Could you check a few things on this drawing? It's one solid part, dimensions in mm from its lowest x, y, z. Round coordinates to 2 decimals unless told otherwise and drop trailing zeros. Write each loop counter-clockwise with the first axis right and the second up, starting at its lowest first coordinate (ties: lowest second). Pieces come first, ordered by that corner, then holes. Notation, with made-up numbers: (48, 34.5) - (105, 34.5) arc R21 ccw to (105, 48.5) - close; hole circle Ø9 at (45.25, -1). An arc over 180 degrees is marked (long way). One line per question, with ' | ' between items. Start each with the question number.
(1) Imagine slicing it at C-C (z = 6.75). Write out the boundary of the cut face in (x, y), plus the area to 3 significant figures.
(2) Will these pins go through, and if not, where does the flat tip stop? pin 1 (1.5 mm diameter, centred on y = 6.5, z = 4, fed in from -X); pin 2 (4 mm diameter, centred on y = 5, z = 3.5, fed in from +X); pin 3 (3.5 mm diameter, centred on x = 4, y = 4, fed in from -Z).
(3) Imagine slicing it at D-D (x = 1.75). Write out the boundary of the cut face in (y, z), plus the area to 3 significant figures.
(4) Thinking about a two-plate mould opening in Y: for the marked faces 1, 2 and 3, which applies, pulls with the +Y half, pulls with the -Y half, needs draft (parallel to the pull), parting line crosses it, or undercut?
(5) If I drill on L1, parallel to Y at x = 4, z = 4.5; L2, parallel to Z at x = 7.25, y = 5.75; L3, parallel to Y at x = 3.5, z = 9.5, over which ranges is the centre line in solid material (lowest first)?
(6) Imagine slicing it at A-A (y = 4). Write out the boundary of the cut face in (x, z).
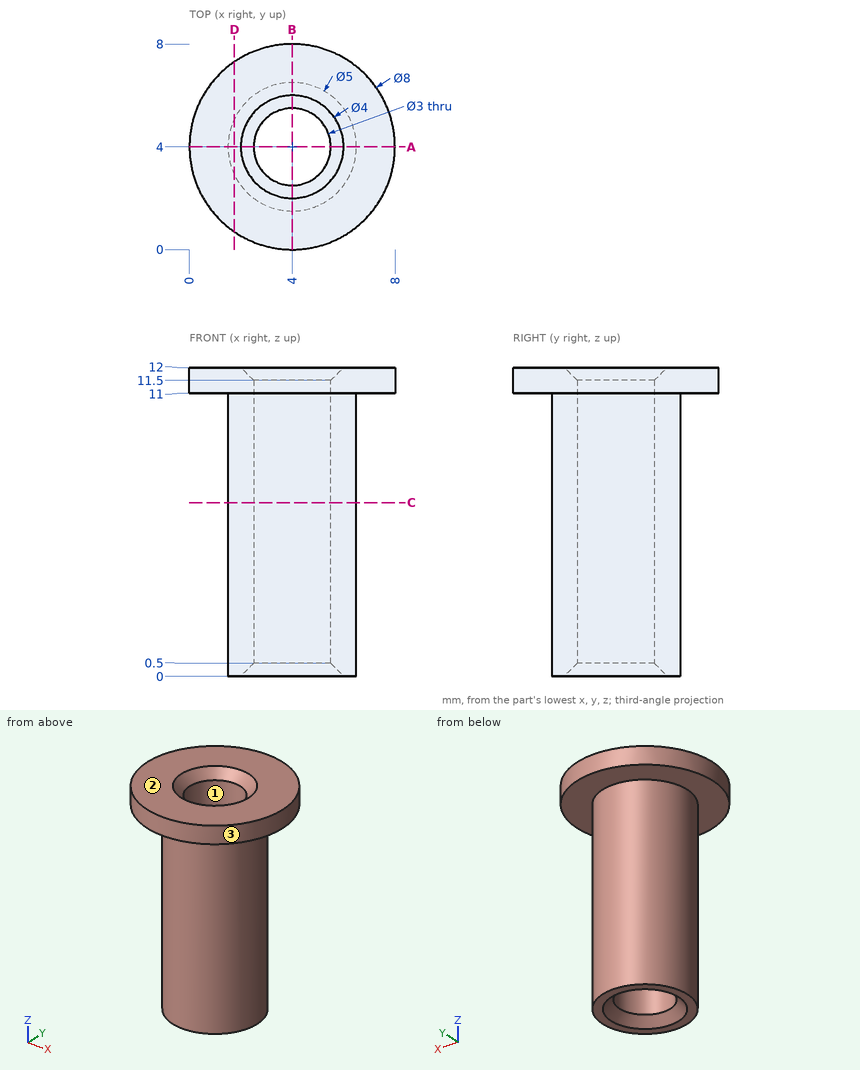
Check sheet entries:
1) outline: circle Ø5 at (4, 4); hole circle Ø3 at (4, 4) | area: 12.6 mm^2
2) pin 1: x = 2.21 | pin 2: x = 6.5 | pin 3: z = 0.25
3) outline: (0.69, 11) - (2.91, 11) - (2.91, 0) - (5.09, 0) - (5.09, 11) - (7.31, 11) - (7.31, 12) - (0.69, 12) - close | area: 30.6 mm^2
4) face 1: undercut | face 2: needs draft | face 3: parting line crosses it
5) L1: 1.5 to 2.5, 5.5 to 6.5 | L2: 11 to 12 | L3: 1.55 to 2.59, 5.41 to 6.45
6) outline: (0, 11) - (1.5, 11) - (1.5, 0) - (2, 0) - (2.5, 0.5) - (2.5, 11.5) - (2, 12) - (0, 12) - close; (5.5, 0.5) - (6, 0) - (6.5, 0) - (6.5, 11) - (8, 11) - (8, 12) - (6, 12) - (5.5, 11.5) - close
